Input: part model. Units: mm. Frame: model coordinates. A direction names the side the tool comes from. Give positions to 0.01 mm unless a question says otherwise; leave off trailing zeros. Write each loop counter-clockwise with the first axis right and the second up, starting at its lowest first coordinate (ties: lowest second). Pieces come first, ordered by that corner, then holes. Notation, with made-up numbers: (75, -36) - (118, -36) arc R10 ccw to (118, -24) - close; hole circle Ø6 at (23, 77). An arc over 180 degrees is marked (long way). Answer as CSV lines item,"result".
```python
from build123d import *

# Parameters (mm, degrees)
F0_W     = 38.1
F0_H     = 38.1
F1_DEPTH = 38.1
F5_DEPTH = 38.1


with BuildPart() as f1:
    # F0 (on Front) → F1 (new body)
    with BuildSketch(Plane.XZ):
        with Locations((19.05, 19.05)):
            Rectangle(F0_W, F0_H)
    extrude(amount=F1_DEPTH)

    # F4 (on offset) → F5 (cut)
    with BuildSketch(Plane.XZ.offset(38.1)):
        Polygon((11.43, 21.469494), (6.35, 0), (31.75, 0), (26.67, 22.225), (21.59, 9.525), (16.51, 9.525), align=None)
        Polygon((31.75, 38.1), (38.1, 0), (38.1, 38.1), align=None)
        Polygon((25.4, 38.1), (12.7, 38.1), (19.05, 22.225), align=None)
        Polygon((6.35, 38.1), (0, 38.1), (0, 0), align=None)
    extrude(amount=-F5_DEPTH, mode=Mode.SUBTRACT)


solid = f1.part
```
Item 1: Cut plane D-D on z = 26.5. Return the cut outline in (x, y), plus the area to 3 significant figures.
The answers:
outline,"(4.42, -38.1) - (17.34, -38.1) - (17.34, 0) - (4.42, 0) - close; (20.76, -38.1) - (33.68, -38.1) - (33.68, 0) - (20.76, 0) - close"
area,"985 mm²"
Item 2: Mould query, pull axis X, two halves, no side actions, for faces 4 (the face through (24.166, -19.317, 15.964)), 5 (the face through (22.2, -19.3, 30.1)), 6 (the face through (19, 0, 19)), 7 (the face through (3.13, -19.32, 18.78)). Classes: +X half, -X half, draft (parallel to the pull), parting line (faces both ways), or undercut.
The answers:
face 4,"undercut"
face 5,"undercut"
face 6,"draft"
face 7,"-X half"
Item 3: Cut plane C-C on z = 12.5. Return the cut outline in (x, y).
The answers:
outline,"(2.08, -38.1) - (9.31, -38.1) - (9.31, 0) - (2.08, 0) - close; (15.24, -38.1) - (22.78, -38.1) - (22.78, 0) - (15.24, 0) - close; (28.89, -38.1) - (36.02, -38.1) - (36.02, 0) - (28.89, 0) - close"
Item 4: Cut plane A-A on z = 33. Return the cut outline in (x, y), plus the area to 3 significant figures.
The answers:
outline,"(5.5, -38.1) - (14.74, -38.1) - (14.74, 0) - (5.5, 0) - close; (23.36, -38.1) - (32.6, -38.1) - (32.6, 0) - (23.36, 0) - close"
area,"704 mm²"
Item 5: Contact query for flat-ended pins moving along their axis: pin 1 (5 mm diameter, centred on y = -7.5, z = 6.5, fed in from +X); pin 2 (2 mm diameter, centred on x = 19.5, y = -8.5, fed in from +Z); pin 3 (8 mm diameter, centred on y = -25.5, z = 22, fed in from -X); pin 4 (3 mm diameter, centred on x = 14, z = 9, fed in from -Y). Output: stop coordinate, or through.
The answers:
pin 1,"x = 37.43"
pin 2,"z = 25.85"
pin 3,"x = 3"
pin 4,"through"
Item 6: Ray query, line 1 (X direction, y = -26, z = 18); line 2 (X direction, y = -23, z = 11.5); line 3 (X direction, y = -14, z = 24.5). Return the intervals inside material, ascending. Write a range as from..to.
The answers:
line 1,"3..10.61, 12.91..24.98, 27.64..35.1"
line 2,"1.92..9.07, 15.67..22.38, 29.12..36.18"
line 3,"4.08..18.14, 19.96..34.02"
Item 7: Reachability of faces 1 (the face through (15.83, -19.32, 30.27)), 2 (the face through (29, -19, 38.1)), 3 (the face through (14.006, -19.317, 15.414)) from +Z, -Z, +X, -X, +Y, -Y: full face, straight path, thin tool, end or side. Return the list, or none.
The answers:
face 1,"+Z, +Y, -Y"
face 2,"+Z, +X, -X, +Y, -Y"
face 3,"-Z, +Y, -Y"
